Geometry: final body of the model. Coordinates: model frame, mm. A direction names the side the tool comes from. Give positions to 0.01 mm unless a question says otherwise; leave off trailing zeros. Write each loop counter-clockwise with the first axis right and the second up, starting at its lowest first coordinate (ties: lowest second). Pieces come first, ordered by that corner, then holes.
```python
from build123d import *

# Parameters (mm, degrees)
SKETCH1_W           = 76.2
SKETCH1_H           = 50.8
BOSS_EXTRUDE1_DEPTH = 6.35
SKETCH2_W           = 50.8
SKETCH2_H           = 25.4
BOSS_EXTRUDE2_DEPTH = 12.7
SKETCH3_R           = 12.7
CUT_EXTRUDE1_DEPTH  = 79.545162168


with BuildPart() as part:
    # Sketch1 → Boss-Extrude1 (new body)
    with BuildSketch(Plane(origin=(0, 0, 0), x_dir=(1, 0, 0), z_dir=(0, 1, 0))):
        Rectangle(SKETCH1_W, SKETCH1_H)
    extrude(amount=BOSS_EXTRUDE1_DEPTH)

    # Sketch2 → Boss-Extrude2 (add, symmetric)
    with BuildSketch(Plane.XY):
        with BuildLine():
            ThreePointArc((-25.4, 31.75), (0, 57.15), (25.4, 31.75))
            Line((25.4, 31.75), (-25.4, 31.75))
        make_face()
        with Locations((0, 19.05)):
            Rectangle(SKETCH2_W, SKETCH2_H)
    extrude(amount=BOSS_EXTRUDE2_DEPTH, both=True)

    # Sketch3 → Cut-Extrude1 (cut, through all)
    with BuildSketch(Plane.XY.offset(12.7)):
        with Locations((0, 31.75)):
            Circle(SKETCH3_R)
    extrude(amount=-CUT_EXTRUDE1_DEPTH, mode=Mode.SUBTRACT)


solid = part.part
```
Item 1: Line query: L1, parallel to X at y = 31, z = 0; L2, parallel to Y at x = 0, z = 5; L3, parallel to X at y = 18, z = 8. Output: solid intervals per line, ascending.
Found:
L1: x = -25.4 to -12.68, 12.68 to 25.4
L2: y = 0 to 19.05, 44.45 to 57.15
L3: x = -25.4 to 25.4
Item 2: Reachability of faces 1 (the face through (12, 26, 12.7)), 2 (the face through (12, 26, -12.7)), 3 (the face through (-25.4, 19, 0)) from +Z, -Z, +X, -X, +Y, -Y: full face, straight path, thin tool, end or side. Return the list, or none.
Found:
face 1: +Z, +X, -X, +Y
face 2: -Z, +X, -X, +Y
face 3: +Z, -Z, -X, +Y
Item 3: Section B-B, the plane x = 0. Return the cut outline in (y, z).
Found:
outline: (0, -25.4) - (6.35, -25.4) - (6.35, -12.7) - (19.05, -12.7) - (19.05, 12.7) - (6.35, 12.7) - (6.35, 25.4) - (0, 25.4) - close; (44.45, -12.7) - (57.15, -12.7) - (57.15, 12.7) - (44.45, 12.7) - close
Item 4: Section A-A, the plane z = 9.5. Return the cut outline in (x, y).
Found:
outline: (-38.1, 0) - (38.1, 0) - (38.1, 6.35) - (25.4, 6.35) - (25.4, 31.75) arc R25.4 ccw to (-25.4, 31.75) - (-25.4, 6.35) - (-38.1, 6.35) - close; hole circle Ø25.4 at (0, 31.75)
Item 5: Pin query (flat end, axial travel): pin 1 Ø3 at (x, z) = (13, 3) entering from +Y; pin 2 Ø8 at (y, z) = (19, -6) entering from +X; pin 3 Ø2 at (y, z) = (19, 5.5) entering from -X; pin 4 Ø1.5 at (x, y) = (-26.5, 22.5) entering from -Z. Return the tip coordinate at first contact, or that it passes through.
Found:
pin 1: stops at y = 54.4
pin 2: stops at x = 25.4
pin 3: stops at x = -25.4
pin 4: passes through
Item 6: Section C-C, the plane y = 23. Return the cut outline in (x, z).
Found:
outline: (-25.4, -12.7) - (-9.2, -12.7) - (-9.2, 12.7) - (-25.4, 12.7) - close; (9.2, -12.7) - (25.4, -12.7) - (25.4, 12.7) - (9.2, 12.7) - close
Item 7: Section D-D, the plane x = -10.5. Return the cut outline in (y, z), plus the area to 3 significant figures.
Found:
outline: (0, -25.4) - (6.35, -25.4) - (6.35, -12.7) - (24.61, -12.7) - (24.61, 12.7) - (6.35, 12.7) - (6.35, 25.4) - (0, 25.4) - close; (38.89, -12.7) - (54.88, -12.7) - (54.88, 12.7) - (38.89, 12.7) - close
area: 1,190 mm2
